Model file for the job. Use its own axes, mm. A direction names the side the tool comes from. Coordinates: 2 decimals unless noted, no trailing zeros. Loops run counter-clockwise (first coordinate to the right, second up) from the corner with the lowest first, then second, coordinate; pieces in that order, holes last.
from build123d import *

# Parameters (mm, degrees)
BOSS_EXTRUDE1_DEPTH = 5.9
FILLET1_R           = 2
FILLET2_R           = 1


with BuildPart() as part:
    # Sketch1 → Boss-Extrude1 (new body)
    with BuildSketch(Plane.XY):
        Polygon((0, 0), (6.95, 0), (6.95, -5.9), (8.95, -5.9), (8.95, -60.9), (-18, -5.9), (0, -5.9), align=None)
        Polygon((-9.982011135, -10.9), (3.95, -10.9), (3.95, -39.332675786), align=None, mode=Mode.SUBTRACT)
    extrude(amount=BOSS_EXTRUDE1_DEPTH)

    # Fillet1
    fillet1_edges = [part.edges().sort_by_distance(p)[0] for p in [
        (8.95, -60.9, 2.95),
    ]]
    fillet(fillet1_edges, radius=FILLET1_R)

    # Fillet2
    fillet2_edges = [part.edges().sort_by_distance(p)[0] for p in [
        (-9.982011135, -10.9, 2.95),
        (3.95, -39.332675786, 2.95),
        (3.95, -10.9, 2.95),
    ]]
    fillet(fillet2_edges, radius=FILLET2_R)


solid = part.part
Q1. Drill centre lines: line 1 (X direction, y = -18.5, z = 4.75); line 2 (Y direction, x = 3.75, z = 2.2); line 3 (Y direction, x = -5.25, z = 4). Where is each one in solid material? Low to high.
Answers:
line 1: x = -11.83 to -6.26, 3.95 to 8.95
line 2: y = -50.29 to -35.62, -11.3 to 0
line 3: y = -31.92 to -20.56, -10.9 to -5.9
Q2. Slice it at C-C (y = -27.5). List the corners of the cut face in (x, z).
Answers:
outline: (-7.42, 0) - (-1.85, 0) - (-1.85, 5.9) - (-7.42, 5.9) - close; (3.95, 0) - (8.95, 0) - (8.95, 5.9) - (3.95, 5.9) - close
Q3. Slice it at A-A (z = 2.05). List the corners of the cut face in (x, y), and give its area (3 significant figures).
Answers:
outline: (-18, -5.9) - (5.15, -53.15) arc R2 ccw to (8.95, -52.27) - (8.95, -5.9) - (6.95, -5.9) - (6.95, 0) - (0, 0) - (0, -5.9) - close; hole (-9.28, -12.34) - (2.05, -35.46) arc R1 ccw to (3.95, -35.02) - (3.95, -11.9) arc R1 ccw to (2.95, -10.9) - (-8.38, -10.9) arc R1 ccw to start
area: 576 mm2
Q4. Mould opens along Y. For faces 1 (the flat face through (8, -5.9, 3)), 2 (the flat face through (-3.533, -24.061, 2.909)), 3 (the cylindrical face through (7.36, -54.23, 2.99)) say: +Y half, -Y half, draft (parallel to the pull), parting line (faces both ways), or undercut.
Answers:
face 1: +Y half
face 2: undercut
face 3: -Y half
Q5. Slice it at B-B (x = 1). List the corners of the cut face in (y, z), and give its area (3 significant figures).
Answers:
outline: (-44.68, 0) - (-33.31, 0) - (-33.31, 5.9) - (-44.68, 5.9) - close; (-10.9, 0) - (0, 0) - (0, 5.9) - (-10.9, 5.9) - close
area: 131 mm2
Q6. Flat gauge pins, fed straight in: P1, Ø1.5, axis at x = -14, z = 3.5, coming from the +Y side; P2, Ø3, axis at x = -3.5, z = 3.5, coming from the -Y side; P3, Ø3, axis at x = -0.5, y = -22.5, coming from the +Z side; P4, Ø3, axis at y = -25.5, z = 3, coming from the -X side. Where does each tip first touch, or does it go through?
Answers:
P1: stops at y = -5.9
P2: stops at y = -38.55
P3: passes through
P4: stops at x = -9.13
Q7. Slice it at D-D (y = -3.5). List the corners of the cut face in (x, z).
Answers:
outline: (0, 0) - (6.95, 0) - (6.95, 5.9) - (0, 5.9) - close
Q8. Which spindle directions (+Z, -Z, +X, -X, +Y, -Y) get a long thin tool onto all of the face, cutting with end or side? Do faces 4 (the flat face through (3, 0, 3)), 5 (the cylindrical face through (-9.22, -11.36, 2.99)), 6 (the flat face through (-4, -27, 5.9)), 7 (the flat face through (6.95, -3, 3)), 8 (the flat face through (0, -3, 3)). Say none if no direction does.
Answers:
face 4: +Z, -Z, +X, -X, +Y
face 5: +Z, -Z
face 6: +Z, +X, -X, +Y, -Y
face 7: +Z, -Z, +X, +Y
face 8: +Z, -Z, -X, +Y
